Input: part model. Units: mm. Frame: model coordinates. Face numbers are marked on the shaded views. Round coordinates to 2 decimals unless told otherwise and drop trailing zeros. Loops run counter-clockwise (first coordinate to the right, second up) from the corner with the lowest first, then second, coordinate; pieces in that order, holes last. Notation, with made-up numbers: (13, 19.25) -> (67, 19.25) arc R26 ccw to (67, 42.25) -> close; hole circle Ø6 at (87.25, -2.5). An arc over 180 degrees is marked (long way). Answer in a Markdown table with one row per item. Add a question column.
Q1. Mould query, pull axis X, two halves, no side actions, for the marked faces 1, 2 and 3. Classes: pulls with the +X half, pulls with the -X half, needs draft (parallel to the pull), parting line crosses it, or undercut.
Q2. Section D-D, the plane y = 14.5. Output: boundary loops of the cut face in (x, z), and give its area (3 significant figures).
Q3. Pin query (flat end, axial travel): pin 1 (1.5 mm diameter, centred on y = 1, z = 4, fed in from -X); pin 2 (6 mm diameter, centred on y = 10, z = 8.5, fed in from +X); pin 3 (8 mm diameter, centred on x = -8, y = -1.5, fed in from -Z); pin 4 (2 mm diameter, centred on x = -5.5, y = -11.5, fed in from -Z). Return the tip coordinate at first contact, or that it passes through.
Q4. Section A-A, the plane y = 0. Output: boundary loops of the cut face in (x, z).
Q5. Section C-C, the plane x = -8.5. Output: boundary loops of the cut face in (y, z).
Q6. Ray query, L1, parallel to X at y = 0, z = 3.75; L2, parallel to X at y = -1.5, z = 0.5; L3, parallel to Y at x = 19, z = 7.5. Return the intervals inside material, ascending. Write a range as from..to.
Q7. Section B-B, the plane z = 4. Output: boundary loops of the cut face in (x, y), and give its area (3 significant figures).
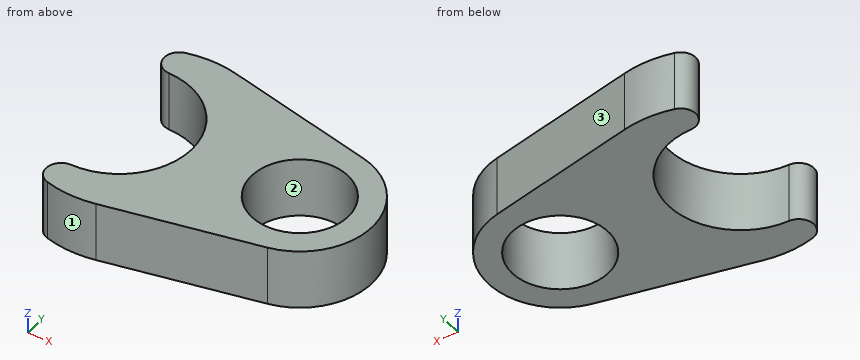
Autodesk Inventor part; units mm, degrees
ref_plane "YZ Plane" through (0, 0, 0) normal (1, 0, 0) x (0, 1, 0)
ref_plane "XZ Plane" through (0, 0, 0) normal (0, 1, 0) x (-1, 0, 0)
ref_plane "XY Plane" through (0, 0, 0) normal (0, 0, 1) x (1, 0, 0)
sketch "스케치1" plane through (0, 0, 0) normal (0, 0, 1) x (1, 0, 0)
  line L0 (0, 41.7955) -> (0, -35.3319)
  line L1 (-51.4236, 0) -> (57.1089, 0)
  arc A0 (-13.077, -11.9993) -> (-13.077, 11.9993) centre (-13.2063, 0) ccw
  circle A1 centre (16.7937, 0) radius 8
  line L2 (19.3321, 11.7284) -> (-5.5044, 17.104)
  line L3 (19.3321, -11.7284) -> (-5.5044, -17.104)
  arc A2 (-13.6907, 16.9157) -> (-13.077, 11.9993) centre (-13.0501, 14.4992) ccw
  arc A3 (-13.077, -11.9993) -> (-13.6907, -16.9157) centre (-13.0501, -14.4992) ccw
  arc A4 (19.3321, -11.7284) -> (19.3321, 11.7284) centre (16.7937, 0) ccw
  arc A5 (-5.5044, 17.104) -> (-13.6907, 16.9157) centre (-9.2063, 0) ccw
  arc A6 (-13.6907, -16.9157) -> (-5.5044, -17.104) centre (-9.2063, 0) ccw
  point P0 (0, 0)
  dimension "d1" = 24
  dimension "d4" = 30
  dimension "d8" = 16
  dimension "d9" = 4
  dimension "d10" = 5
  dimension "d11" = 5
extrude "돌출1" add sketch "스케치1" along normal blind 10 contours L2 A4 L1 A1 L0 | L0 L1 A0 A2 A5 L2 | L1 A1 A4 L3 L0 | L0 L3 A6 A3 A0 L1
properties part number "240412_sketch4"
Answer block:
| question | item | result |
|---|---|---|
| 1 | face 1 | parting line crosses it |
| 1 | face 2 | undercut |
| 1 | face 3 | pulls with the +X half |
| 2 | outline | (-15.55, 0) -> (6.53, 0) -> (6.53, 10) -> (-15.55, 10) -> close |
| 2 | area | 221 mm^2 |
| 3 | pin 1 | x = -1.33 |
| 3 | pin 2 | x = 26.54 |
| 3 | pin 3 | through |
| 3 | pin 4 | z = 0 |
| 4 | outline | (-1.21, 0) -> (8.79, 0) -> (8.79, 10) -> (-1.21, 10) -> close; (24.79, 0) -> (28.79, 0) -> (28.79, 10) -> (24.79, 10) -> close |
| 5 | outline | (-17.49, 0) -> (-11.04, 0) -> (-11.04, 10) -> (-17.49, 10) -> close; (11.04, 0) -> (17.49, 0) -> (17.49, 10) -> (11.04, 10) -> close |
| 6 | L1 | -1.21..8.79, 24.79..28.79 |
| 6 | L2 | -1.3..8.94, 24.65..28.7 |
| 6 | L3 | -11.8..-7.69, 7.69..11.8 |
| 7 | outline | (-13.69, -16.92) arc R17.5 ccw to (-5.5, -17.1) -> (19.33, -11.73) arc R12 ccw to (19.33, 11.73) -> (-5.5, 17.1) arc R17.5 ccw to (-13.69, 16.92) arc R2.5 ccw to (-13.08, 12) arc R12 cw to (-13.08, -12) arc R2.5 ccw to start; hole circle Ø16 at (16.79, 0) |
| 7 | area | 740 mm^2 |
